CAD build for the part. Positions are in the model's coordinates, mm. A direction names the side the tool comes from. Coordinates: 2 decimals unless noted, no trailing zeros. Order: outer loops, then holes, each group sorted by start corner. A loop starts at its lowest first (then second) coordinate and runs counter-clockwise, first axis right, second up. Notation, with made-up numbers: M -20.75,11.25 L 3.25,11.25 A21 cw 3.25,27.25 Z; hole C -14,68 d10. An arc over 180 degrees is marked long. Write item = value, one per line.
Autodesk Inventor part; units mm, degrees
ref_plane "Work Plane1" through (0, 9.15, 0) normal (0, 1, 0) x (-1, 0, 0)
ref_plane "Work Plane4" through (34.15, 0, 0) normal (1, 0, 0) x (0, 1, 0)
ref_plane "XY Plane" through (0, 0, 0) normal (0, 0, 1) x (1, 0, 0)
sketch "Sketch1" plane through (0, 0, 0) normal (0, 0, 1) x (1, 0, 0)
  circle A0 centre (0, 0) radius 3.7
  circle A1 centre (0, 0) radius 9.15
  dimension "d0" = 7.4
  dimension "d1" = 18.3
extrude "Extrusion1" add sketch "Sketch1" along normal mid plane 30
ref_plane "Work Plane1" through (0, 9.15, 0) normal (0, 1, 0) x (-1, 0, 0)
ref_plane "Work Plane2" through (-9.15, 0, 0) normal (1, 0, 0) x (0, 1, 0)
ref_plane "Work Plane4" through (34.15, 0, 0) normal (1, 0, 0) x (0, 1, 0)
ref_plane "Work Plane3" through (9.15, 0, 0) normal (1, 0, 0) x (0, 1, 0)
sketch "Sketch2" plane through (-9.15, 5.7, 0) normal (1, 0, 0) x (0, 1, 0)
  point P0 (-5.7, 0)
  point P1 (-5.7, 0)
hole "Hole1" at (-9.15, 0, 0) direction (1, 0, 0) diameter 2 depth 3
sketch "Sketch4" plane through (34.15, 0, 0) normal (1, 0, 0) x (0, 1, 0)
  circle A0 centre (0, 0) radius 9.15
  circle A1 centre (0, 0) radius 7.15
  dimension "d19" = 14.3
  dimension "d20" = 18.3
extrude "Bottom Extrusion" add sketch "Sketch4" against normal up to surface
sketch "Sketch6" plane through (0, 9.15, 0) normal (0, 1, 0) x (-1, 0, 0)
  line L0 (0, 0) -> (-31, 0) construction
  point P0 (-15.5, 0)
hole "Hole2" at (15.5, 9.15, 0) direction (0, -1, 0) diameter 2 end through all
extrude "Cut for wire" cut sketch "Sketch4" against normal blind 34 contours A1
properties part number "Part6_3DPrint"
(1) Pull direction Z, two halves, no side cores. Call faces 1 (the face through (-6.15, 0, 0)), 2 (the face through (16.476, 8.1, -0.217)), 3 (the face through (4, 0, -15)), 4 (the face through (-3.696, -0.163, -0.21)): +Z half, -Z half, draft (parallel to the pull), parting line (faces both ways), or undercut.
Evaluation:
face_1 = undercut
face_2 = undercut
face_3 = -Z half
face_4 = draft
(2) Slice it at B-B, the plane z = -12. Write the cut outline in (x, y).
Evaluation:
outline = C 0,0 d18.3; hole C 0,0 d7.4
(3) Tool access for faces 5 (the face through (16.476, -8.129, -0.217)), 6 (the face through (34.15, -6.14, -4.02)), 7 (the face through (0.15, -5, 0)), 8 (the face through (-8, 1, 0)), 9 (the face through (-6.744, -6.184, -0.21)): list every direction of +Z, -Z, +X, -X, +Y, -Y with a clear straight run to the whole face (end or side of a thin tool).
Evaluation:
face_5 = +Y, -Y
face_6 = +Z, -Z, +X, +Y, -Y
face_7 = +X
face_8 = -X
face_9 = none
(4) Slice it at C-C, the plane x = 27.5. Write the cut outline in (y, z).
Evaluation:
outline = C 0,0 d18.3; hole C 0,0 d14.3
(5) Slice it at D-D, the plane z = -4.5. Write the cut outline in (x, y), then the cut area to 3 significant figures.
Evaluation:
outline = M 0.15,-5.56 L 0.15,-3.7 A3.7 cw long 0.15,3.7 L 0.15,5.56 L 34.15,5.56 L 34.15,7.97 L 4.5,7.97 A9.15 ccw long 4.5,-7.97 L 34.15,-7.97 L 34.15,-5.56 Z
area = 282 mm²
(6) Wall check: line 1 (Z direction, x = 16, y = 0); line 2 (Z direction, x = 9, y = -1); line 3 (X direction, y = 7.8, z = 0). Give the ranges that are in metal, low to high. Write a range as from..to.
Evaluation:
line_1 = -9.15..-7.15, 7.15..9.15
line_2 = -15..-7.08, 7.08..15
line_3 = -4.78..14.5, 16.5..34.15
(7) Slice it at A-A, the plane y = 0. Write the cut outline in (x, z), then the cut area to 3 significant figures.
Evaluation:
outline = M -9.15,-15 L -3.7,-15 L -3.7,15 L -9.15,15 L -9.15,1 L -6.15,1 L -6.15,-1 L -9.15,-1 Z; M 3.7,-15 L 9.15,-15 L 9.15,-9.15 L 34.15,-9.15 L 34.15,-7.15 L 3.7,-7.15 Z; M 3.7,7.15 L 34.15,7.15 L 34.15,9.15 L 9.15,9.15 L 9.15,15 L 3.7,15 Z
area = 343 mm²
(8) Pin check, flat tips, straight feed: pin 1 Ø1.5 at (x, y) = (19, 4) entering from -Z; pin 2 Ø1 at (y, z) = (-5.5, -3) entering from +X; pin 3 Ø2.5 at (x, z) = (15.5, 0) entering from -Y; pin 4 Ø1 at (x, y) = (28, -2) entering from -Z. Stop position of each tip, or through.
Evaluation:
pin_1 = -8.55
pin_2 = 0.15
pin_3 = -9.15
pin_4 = -9.03
